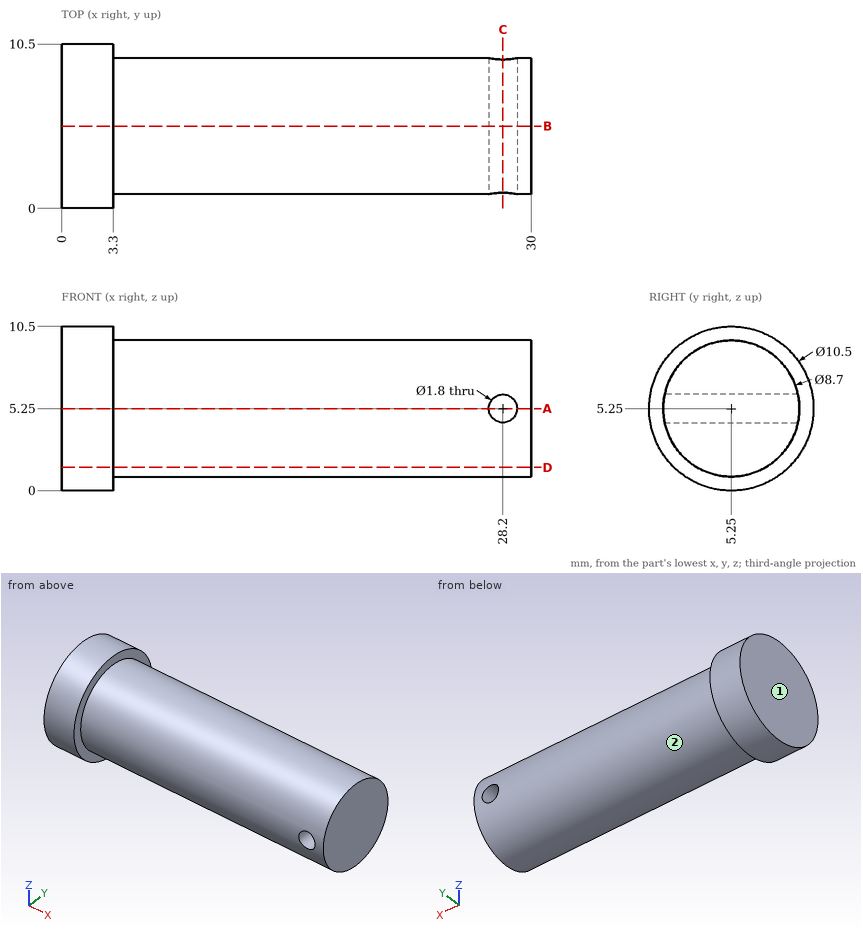
The drawing under review shows one solid part. Ordinate dimensions are in mm from its lowest x, y, z. A direction names the side the tool comes from. Round coordinates to 2 decimals unless told otherwise and drop trailing zeros. Order: outer loops, then holes, each group sorted by start corner. A loop starts at its lowest first (then second) coordinate and runs counter-clockwise, first axis right, second up. Notation, with made-up numbers: M 27.25,-19.5 L 70.25,-19.5 A16 cw 70.25,2.5 Z; hole C 9,-33.75 d1. An arc over 180 degrees is marked long. Answer as CSV lines item,"result". Start each with the question number.
1) Wall thickness on line 1 along X through (y, z) = (6, 5.25); line 2 along Z through (x, y) = (19, 5); line 3 along X through (y, z) = (7, 5.75): over which ranges is each line inside the solid? List them lowest first. Write a range as [from, to].
2) Add section C-C (x = 28.2). Give the boundary of the cut face in (y, z).
3) Add section A-A (z = 5.25). Give the boundary of the cut face in (x, y), then the cut area to 3 significant figures.
4) For pin 1 Ø2.5 at (x, z) = (28.2, 5.25) entering from -Y; pin 2 Ø2 at (x, z) = (4, 5.5) entering from -Y; pin 3 Ø1 at (x, y) = (24.5, 4.5) entering from -Z, all flat-tipped, find the tip position at first contact; note any pin that passes through.
5) Tool access review of the marked faces 1 and 2: name each direction out of +Z, -Z, +X, -X, +Y, -Y from which nothing blocks a thin tool from reaching the whole face with its end or side.
6) Add section B-B (y = 5.25). Give the boundary of the cut face in (x, z), then the cut area to 3 significant figures.
7) Add section D-D (z = 1.5). Give the boundary of the cut face in (x, y).
Resolved:
1,line 1,"[0, 27.3], [29.1, 30]"
1,line 2,"[0.91, 9.59]"
1,line 3,"[0, 27.45], [28.95, 30]"
2,outline,"M 0.99,4.35 A4.35 ccw 9.51,4.35 Z; M 0.99,6.15 L 9.51,6.15 A4.35 ccw Z"
3,outline,"M 0,0 L 3.3,0 L 3.3,0.9 L 27.3,0.9 L 27.3,9.6 L 3.3,9.6 L 3.3,10.5 L 0,10.5 Z; M 29.1,0.9 L 30,0.9 L 30,9.6 L 29.1,9.6 Z"
3,area,"251 mm^2"
4,pin 1,"y = 0.9"
4,pin 2,"y = 0"
4,pin 3,"z = 0.91"
5,face 1,"+Z, -Z, -X, +Y, -Y"
5,face 2,"+X"
6,outline,"M 0,0 L 3.3,0 L 3.3,0.9 L 30,0.9 L 30,9.6 L 3.3,9.6 L 3.3,10.5 L 0,10.5 Z; hole C 28.2,5.25 d1.8"
6,area,"264 mm^2"
7,outline,"M 0,1.58 L 3.3,1.58 L 3.3,3.05 L 30,3.05 L 30,7.45 L 3.3,7.45 L 3.3,8.92 L 0,8.92 Z"
